The model under review builds one solid part; all positions refer to its coordinate system, in mm. Face numbers are marked on the shaded views. Round coordinates to 2 decimals unless told otherwise and drop trailing zeros. Write each loop counter-clockwise with the first axis right and the second up, starting at its lowest first coordinate (ties: lowest second). Pieces come first, ordered by that corner, then holes.
Item 1: Add section B-B (y = -29). Give the boundary of the cut face in (x, z).
Item 2: Add section A-A (x = 0). Give the boundary of the cut face in (y, z) (1 decimal).
Item 3: Add section C-C (z = 2.5). State how many separate pieces and enclosed holes the cut face has, plus the area to 3 significant figures.
Item 4: To check wall thickness, follow L1, parallel to Y at x = 0, z = 3 (1 decimal); L2, parallel to Y at x = -16.5, z = 1; L3, parallel to Y at x = 16, z = 0.75. State the ranges of each line that lie inside material, in increasing order.
Item 5: Clearance check with flat-ended pins moving along their axes: pin 1 Ø13.5 at (x, y) = (0, 0) entering from +Z; pin 2 Ø1.5 at (x, z) = (-17, 2.5) entering from -Y; pin 3 Ø1 at (y, z) = (-9.5, 6) entering from -X; pin 4 Ø4 at (y, z) = (-26.5, 3) entering from +X. State where each tip first meets the part, or that it passes through.
Item 6: Draft analysis for pull direction X (two halves, no side actions). For the marked faces 1, 2 and 3, state which applies: +X half, -X half, draft (parallel to the pull), parting line (faces both ways), or undercut.
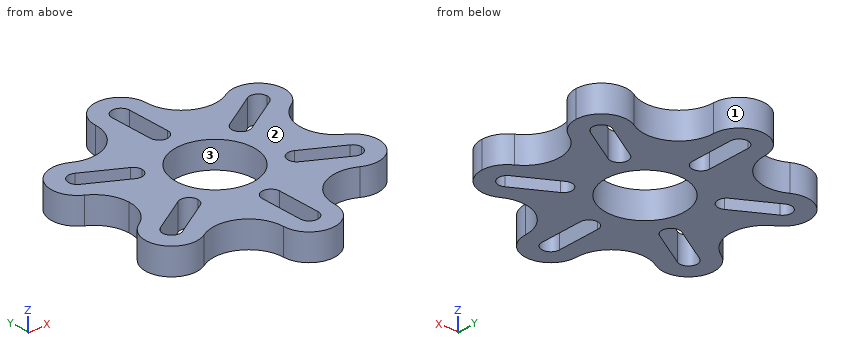
```python
from build123d import *

# Parameters (mm, degrees)
F0_R     = 11.125
F1_DEPTH = 7.5
F3_DEPTH = 25


with BuildPart() as f1:
    # F0 (on Top) → F1 (new body)
    with BuildSketch(Plane.XY):
        with BuildLine():
            ThreePointArc((7.3205080757, 30), (0, 22.6794919243), (-7.3205080757, 30))
            ThreePointArc((-7.3205080757, 30), (-12.3205080803, 21.3397459595), (-22.3205080849, 21.3397459675))
            ThreePointArc((-22.3205080849, 21.3397459675), (-19.641016154, 18.6602540424), (-18.6602540378, 15))
            ThreePointArc((-18.6602540378, 15), (-22.3205080792, 8.6602540358), (-29.6410161584, 8.6602540419))
            ThreePointArc((-29.6410161584, 8.6602540419), (-25.9807621156, 5.0000000035), (-24.6410161514, 0))
            ThreePointArc((-24.6410161514, 0), (-25.9807621131, -4.9999999992), (-29.6410161498, -8.660254037))
            ThreePointArc((-29.6410161498, -8.660254037), (-22.3205080749, -8.6602540383), (-18.6602540378, -15))
            ThreePointArc((-18.6602540378, -15), (-19.6410161418, -18.6602540212), (-22.3205080425, -21.339745943))
            ThreePointArc((-22.3205080425, -21.339745943), (-12.3205080591, -21.3397459717), (-7.3205080757, -30))
            ThreePointArc((-7.3205080757, -30), (0, -22.6794919243), (7.3205080757, -30))
            ThreePointArc((7.3205080757, -30), (12.3205080629, -21.3397459695), (22.3205080502, -21.3397459474))
            ThreePointArc((22.3205080502, -21.3397459474), (19.6410161514, -11.3397459622), (29.6410161259, -8.6602540231))
            ThreePointArc((29.6410161259, -8.6602540231), (24.6410161514, -3.02e-08), (29.6410160736, 8.6602539929))
            ThreePointArc((29.6410160736, 8.6602539929), (19.641016124, 11.3397460095), (22.3205080926, 21.3397459719))
            ThreePointArc((22.3205080926, 21.3397459719), (12.3205080841, 21.3397459573), (7.3205080757, 30))
        make_face()
        Circle(F0_R, mode=Mode.SUBTRACT)
        with BuildLine():
            Line((7.3205080757, 30), (-7.3205080757, 30))
            ThreePointArc((-7.3205080757, 30), (0, 22.6794919243), (7.3205080757, 30))
        make_face()
        with BuildLine():
            ThreePointArc((7.3205080757, 30), (0, 37.3205080757), (-7.3205080757, 30))
            Line((-7.3205080757, 30), (7.3205080757, 30))
        make_face()
        with BuildLine():
            ThreePointArc((-18.6602540378, 15), (-19.641016154, 18.6602540424), (-22.3205080849, 21.3397459675))
            Line((-22.3205080757, 21.3397459622), (-29.6410161514, 8.6602540378))
            ThreePointArc((-29.6410161584, 8.6602540419), (-22.3205080792, 8.6602540358), (-18.6602540378, 15))
        make_face()
        with BuildLine():
            Line((-29.6410161514, 8.6602540378), (-22.3205080757, 21.3397459622))
            ThreePointArc((-22.3205080849, 21.3397459675), (-32.3205080763, 18.6602540368), (-29.6410161584, 8.6602540419))
        make_face()
        with BuildLine():
            ThreePointArc((-18.6602540378, -15), (-22.3205080749, -8.6602540383), (-29.6410161498, -8.660254037))
            Line((-29.6410161514, -8.6602540378), (-22.3205080757, -21.3397459622))
            ThreePointArc((-22.3205080425, -21.339745943), (-19.6410161418, -18.6602540212), (-18.6602540378, -15))
        make_face()
        with BuildLine():
            Line((-22.3205080757, -21.3397459622), (-29.6410161514, -8.6602540378))
            ThreePointArc((-29.6410161498, -8.660254037), (-32.3205080665, -18.6602540537), (-22.3205080425, -21.339745943))
        make_face()
        with BuildLine():
            Line((7.3205080757, -30), (-7.3205080757, -30))
            ThreePointArc((-7.3205080757, -30), (0, -37.3205080757), (7.3205080757, -30))
        make_face()
        with BuildLine():
            ThreePointArc((7.3205080757, -30), (0, -22.6794919243), (-7.3205080757, -30))
            Line((-7.3205080757, -30), (7.3205080757, -30))
        make_face()
        with BuildLine():
            Line((22.3205080757, -21.3397459622), (29.6410161514, -8.6602540378))
            ThreePointArc((29.6410161259, -8.6602540231), (19.6410161514, -11.3397459622), (22.3205080502, -21.3397459474))
        make_face()
        with BuildLine():
            ThreePointArc((33.3012701892, -15), (32.3205080683, -11.3397459494), (29.6410161259, -8.6602540231))
            Line((29.6410161514, -8.6602540378), (22.3205080757, -21.3397459622))
            ThreePointArc((22.3205080502, -21.3397459474), (29.6410161386, -21.3397459695), (33.3012701892, -15))
        make_face()
        with BuildLine():
            Line((29.6410161514, 8.6602540378), (22.3205080757, 21.3397459622))
            ThreePointArc((22.3205080926, 21.3397459719), (19.641016124, 11.3397460095), (29.6410160736, 8.6602539929))
        make_face()
        with BuildLine():
            ThreePointArc((33.3012701892, 15), (29.6410161598, 21.3397459573), (22.3205080926, 21.3397459719))
            Line((22.3205080757, 21.3397459622), (29.6410161514, 8.6602540378))
            ThreePointArc((29.6410160736, 8.6602539929), (32.3205080532, 11.3397459232), (33.3012701892, 15))
        make_face()
    extrude(amount=F1_DEPTH)

    # F2 (on face) → F3 (cut)
    with BuildSketch(Plane.XY.offset(7.5)):
        with BuildLine():
            ThreePointArc((-2.5, 17.8399104625), (0, 15.3399104625), (2.5, 17.8399104625))
            ThreePointArc((2.5, 17.8399104625), (0, 20.3399104625), (-2.5, 17.8399104625))
        make_face()
        with BuildLine():
            Line((2.5, 17.8399104625), (2.5, 30))
            ThreePointArc((2.5, 30), (0, 27.5), (-2.5, 30))
            Line((-2.5, 30), (-2.5, 17.8399104625))
            ThreePointArc((-2.5, 17.8399104625), (0, 20.3399104625), (2.5, 17.8399104625))
        make_face()
        with BuildLine():
            ThreePointArc((-2.5, 30), (0, 27.5), (2.5, 30))
            ThreePointArc((2.5, 30), (0, 32.5), (-2.5, 30))
        make_face()
        with BuildLine():
            ThreePointArc((-24.7307621135, 17.1650635095), (-23.8156986041, 16.25), (-23.4807621135, 15))
            ThreePointArc((-23.4807621135, 15), (-24.7307621135, 12.8349364905), (-27.2307621135, 12.8349364905))
            Line((-27.2307621135, 12.8349364905), (-16.6998156618, 6.7548917218))
            ThreePointArc((-16.6998156618, 6.7548917218), (-17.6148791712, 10.1699552312), (-14.1998156618, 11.0850187407))
            Line((-14.1998156618, 11.0850187407), (-24.7307621135, 17.1650635095))
        make_face()
        with BuildLine():
            ThreePointArc((-12.9498156618, 8.9199552312), (-13.2847521523, 10.1699552312), (-14.1998156618, 11.0850187407))
            ThreePointArc((-14.1998156618, 11.0850187407), (-17.6148791712, 10.1699552312), (-16.6998156618, 6.7548917218))
            ThreePointArc((-16.6998156618, 6.7548917218), (-14.1998156618, 6.7548917218), (-12.9498156618, 8.9199552312))
        make_face()
        with BuildLine():
            ThreePointArc((-27.2307621135, 12.8349364905), (-24.7307621135, 12.8349364905), (-23.4807621135, 15))
            ThreePointArc((-23.4807621135, 15), (-23.8156986041, 16.25), (-24.7307621135, 17.1650635095))
            ThreePointArc((-24.7307621135, 17.1650635095), (-28.145825623, 16.25), (-27.2307621135, 12.8349364905))
        make_face()
        with BuildLine():
            ThreePointArc((-27.2307621135, -12.8349364905), (-24.7307621135, -12.8349364905), (-23.4807621135, -15))
            ThreePointArc((-23.4807621135, -15), (-23.8156986041, -16.25), (-24.7307621135, -17.1650635095))
            Line((-24.7307621135, -17.1650635095), (-14.1998156618, -11.0850187407))
            ThreePointArc((-14.1998156618, -11.0850187407), (-17.6148791712, -10.1699552312), (-16.6998156618, -6.7548917218))
            Line((-16.6998156618, -6.7548917218), (-27.2307621135, -12.8349364905))
        make_face()
        with BuildLine():
            ThreePointArc((-12.9498156618, -8.9199552312), (-14.1998156618, -6.7548917218), (-16.6998156618, -6.7548917218))
            ThreePointArc((-16.6998156618, -6.7548917218), (-17.6148791712, -10.1699552312), (-14.1998156618, -11.0850187407))
            ThreePointArc((-14.1998156618, -11.0850187407), (-13.2847521523, -10.1699552312), (-12.9498156618, -8.9199552312))
        make_face()
        with BuildLine():
            ThreePointArc((-24.7307621135, -17.1650635095), (-23.8156986041, -16.25), (-23.4807621135, -15))
            ThreePointArc((-23.4807621135, -15), (-24.7307621135, -12.8349364905), (-27.2307621135, -12.8349364905))
            ThreePointArc((-27.2307621135, -12.8349364905), (-28.145825623, -16.25), (-24.7307621135, -17.1650635095))
        make_face()
        with BuildLine():
            ThreePointArc((-2.5, -30), (0, -27.5), (2.5, -30))
            Line((2.5, -30), (2.5, -17.8399104625))
            ThreePointArc((2.5, -17.8399104625), (0, -20.3399104625), (-2.5, -17.8399104625))
            Line((-2.5, -17.8399104625), (-2.5, -30))
        make_face()
        with BuildLine():
            ThreePointArc((-2.5, -17.8399104625), (0, -20.3399104625), (2.5, -17.8399104625))
            ThreePointArc((2.5, -17.8399104625), (0, -15.3399104625), (-2.5, -17.8399104625))
        make_face()
        with BuildLine():
            ThreePointArc((-2.5, -30), (0, -32.5), (2.5, -30))
            ThreePointArc((2.5, -30), (0, -27.5), (-2.5, -30))
        make_face()
        with BuildLine():
            ThreePointArc((24.7307621135, -17.1650635095), (23.8156986041, -13.75), (27.2307621135, -12.8349364905))
            Line((27.2307621135, -12.8349364905), (16.6998156618, -6.7548917218))
            ThreePointArc((16.6998156618, -6.7548917218), (17.6148791712, -7.6699552312), (17.9498156618, -8.9199552312))
            ThreePointArc((17.9498156618, -8.9199552312), (16.6998156618, -11.0850187407), (14.1998156618, -11.0850187407))
            Line((14.1998156618, -11.0850187407), (24.7307621135, -17.1650635095))
        make_face()
        with BuildLine():
            ThreePointArc((17.9498156618, -8.9199552312), (17.6148791712, -7.6699552312), (16.6998156618, -6.7548917218))
            ThreePointArc((16.6998156618, -6.7548917218), (13.2847521523, -7.6699552312), (14.1998156618, -11.0850187407))
            ThreePointArc((14.1998156618, -11.0850187407), (16.6998156618, -11.0850187407), (17.9498156618, -8.9199552312))
        make_face()
        with BuildLine():
            ThreePointArc((24.7307621135, -17.1650635095), (27.2307621135, -17.1650635095), (28.4807621135, -15))
            ThreePointArc((28.4807621135, -15), (28.145825623, -13.75), (27.2307621135, -12.8349364905))
            ThreePointArc((27.2307621135, -12.8349364905), (23.8156986041, -13.75), (24.7307621135, -17.1650635095))
        make_face()
        with BuildLine():
            ThreePointArc((27.2307621135, 12.8349364905), (23.8156986041, 13.75), (24.7307621135, 17.1650635095))
            Line((24.7307621135, 17.1650635095), (14.1998156618, 11.0850187407))
            ThreePointArc((14.1998156618, 11.0850187407), (16.6998156618, 11.0850187407), (17.9498156618, 8.9199552312))
            ThreePointArc((17.9498156618, 8.9199552312), (17.6148791712, 7.6699552312), (16.6998156618, 6.7548917218))
            Line((16.6998156618, 6.7548917218), (27.2307621135, 12.8349364905))
        make_face()
        with BuildLine():
            ThreePointArc((17.9498156618, 8.9199552312), (16.6998156618, 11.0850187407), (14.1998156618, 11.0850187407))
            ThreePointArc((14.1998156618, 11.0850187407), (13.2847521523, 7.6699552312), (16.6998156618, 6.7548917218))
            ThreePointArc((16.6998156618, 6.7548917218), (17.6148791712, 7.6699552312), (17.9498156618, 8.9199552312))
        make_face()
        with BuildLine():
            ThreePointArc((27.2307621135, 12.8349364905), (28.145825623, 13.75), (28.4807621135, 15))
            ThreePointArc((28.4807621135, 15), (27.2307621135, 17.1650635095), (24.7307621135, 17.1650635095))
            ThreePointArc((24.7307621135, 17.1650635095), (23.8156986041, 13.75), (27.2307621135, 12.8349364905))
        make_face()
    extrude(amount=-F3_DEPTH, mode=Mode.SUBTRACT)


solid = f1.part
```
Numbers:
1. outline: (-7.37, 0) - (-2.5, 0) - (-2.5, 7.5) - (-7.37, 7.5) - close; (2.5, 0) - (7.37, 0) - (7.37, 7.5) - (2.5, 7.5) - close
2. outline: (-37.3, 0) - (-32.5, 0) - (-32.5, 7.5) - (-37.3, 7.5) - close; (-15.3, 0) - (-11.1, 0) - (-11.1, 7.5) - (-15.3, 7.5) - close; (11.1, 0) - (15.3, 0) - (15.3, 7.5) - (11.1, 7.5) - close; (32.5, 0) - (37.3, 0) - (37.3, 7.5) - (32.5, 7.5) - close
3. separate pieces: 1
3. enclosed holes: 7
3. area: 2,120 mm2
4. L1: y = -37.3 to -32.5, -15.3 to -11.1, 11.1 to 15.3, 32.5 to 37.3
4. L2: y = -20.03 to -12.41, -6.65 to 6.65, 12.41 to 20.03
4. L3: y = -20.09 to -12.12, -6.48 to 6.48, 12.12 to 20.09
5. pin 1: passes through
5. pin 2: stops at y = -20.06
5. pin 3: stops at x = -31.33
5. pin 4: stops at x = 8.97
6. face 1: parting line
6. face 2: draft
6. face 3: undercut
